```python
from build123d import *

# Parameters (mm, degrees)
SKETCH4_W           = 16.730770432
SKETCH4_H           = 61.894764582
SKETCH4_R           = 3.048230072
BOSS_EXTRUDE4_DEPTH = 10
BOSS_EXTRUDE5_DEPTH = 61.894764581
SKETCH6_R           = 3.22777379
CUT_EXTRUDE1_DEPTH  = 301.068940686
CUT_EXTRUDE2_START  = 17.78
SKETCH8_W           = 8.976833554
SKETCH8_H           = 8.976833554
CUT_EXTRUDE2_DEPTH  = 30.32
SKETCH9_R           = 3.75
CUT_EXTRUDE3_DEPTH  = 30.32
SKETCH10_R          = 8.1
CUT_EXTRUDE4_DEPTH  = 20


with BuildPart() as part:
    # Sketch4 → Boss-Extrude4 (new body)
    with BuildSketch(Plane.XY):
        with Locations((241.3, -38.1)):
            Rectangle(SKETCH4_W, SKETCH4_H)
        with Locations((241.3, -12.7)):
            Circle(SKETCH4_R, mode=Mode.SUBTRACT)
        with Locations((241.3, -38.1)):
            Circle(SKETCH4_R, mode=Mode.SUBTRACT)
        with Locations((241.3, -63.5)):
            Circle(SKETCH4_R, mode=Mode.SUBTRACT)
    extrude(amount=BOSS_EXTRUDE4_DEPTH)

    # Sketch5 → Boss-Extrude5 (add)
    with BuildSketch(Plane.XZ.offset(69.047382291)):
        Polygon((249.665385216, 10), (203.509422764, 131.615224448), (203.509422764, 151.462944604), (160.545206695, 151.462944604), (160.545206695, 127.74240556), (188.24848215, 127.74240556), (232.934614784, 10), align=None)
    extrude(amount=-BOSS_EXTRUDE5_DEPTH)

    # Sketch6 → Cut-Extrude1 (cut, through all)
    with BuildSketch(Plane(origin=(0, 0, 0), x_dir=(-1, 0, 0), z_dir=(0, 0, -1))):
        with Locations((-241.3, -63.5)):
            Circle(SKETCH6_R)
        with Locations((-241.3, -38.1)):
            Circle(SKETCH6_R)
        with Locations((-241.3, -12.7)):
            Circle(SKETCH6_R)
    extrude(amount=-CUT_EXTRUDE1_DEPTH, mode=Mode.SUBTRACT)

    # Sketch8 → Cut-Extrude2 (cut)
    with BuildSketch(Plane.XY.offset(CUT_EXTRUDE2_START)):
        with Locations((241.3, -63.5)):
            Rectangle(SKETCH8_W, SKETCH8_H)
        with Locations((241.3, -38.1)):
            Rectangle(SKETCH8_W, SKETCH8_H)
        with Locations((241.3, -12.7)):
            Rectangle(SKETCH8_W, SKETCH8_H)
    extrude(amount=CUT_EXTRUDE2_DEPTH, mode=Mode.SUBTRACT)

    # Sketch9 → Cut-Extrude3 (cut)
    with BuildSketch(Plane.XY.offset(151.462944604)):
        with Locations((182.02731473, -38.1)):
            Circle(SKETCH9_R)
    extrude(amount=-CUT_EXTRUDE3_DEPTH, mode=Mode.SUBTRACT)

    # Sketch10 → Cut-Extrude4 (cut)
    with BuildSketch(Plane.XY.offset(151.462944604)):
        with Locations((182.02731473, -38.1)):
            Circle(SKETCH10_R)
    extrude(amount=-CUT_EXTRUDE4_DEPTH, mode=Mode.SUBTRACT)


solid = part.part
```
Read the model definition and answer for the solid it produces. Units are mm, in the model's axes. A direction names the side the tool comes from. Round coordinates to 2 decimals unless told otherwise and drop trailing zeros. Write each loop counter-clockwise with the first axis right and the second up, starting at its lowest first coordinate (ties: lowest second). Pieces come first, ordered by that corner, then holes. Notation, with made-up numbers: (26.25, 38.25) - (77.25, 38.25) arc R22 ccw to (77.25, 74.25) - close; hole circle Ø3 at (-28.5, -34). An arc over 180 degrees is marked (long way). Use CSV: the item, a comma, the result in double quotes.
Q1. Find section D-D, the plane y = -63.5. Write down the section's boundary in (x, z).
Values:
outline,"(160.55, 127.74) - (188.25, 127.74) - (232.93, 10) - (232.93, 0) - (238.07, 0) - (238.07, 17.78) - (236.81, 17.78) - (236.81, 43.87) - (203.51, 131.62) - (203.51, 151.46) - (160.55, 151.46) - close; (244.53, 0) - (249.67, 0) - (249.67, 10) - (245.79, 20.22) - (245.79, 17.78) - (244.53, 17.78) - close"
Q2. Find section C-C, the plane z = 137.5. Write down the section's boundary in (x, y).
Values:
outline,"(160.55, -69.05) - (203.51, -69.05) - (203.51, -7.15) - (160.55, -7.15) - close; hole circle Ø16.2 at (182.03, -38.1)"
Q3. Each of these flat-tipped pins is pushed along its axis until it touches: pin 1 Ø3 at (y, z) = (-33, 126) entering from +X; pin 2 Ø12 at (x, y) = (182.03, -38.1) entering from -Z; pin 3 Ø3 at (y, z) = (-30.5, 93) entering from -X. Where does it stop, or does it pass through?
Values:
pin 1,"stops at x = 206.21"
pin 2,"stops at z = 127.74"
pin 3,"stops at x = 200.86"
Q4. Determine the mould class of faces 1 (the flat face through (210.279, -38.533, 69.695)), 2 (the flat face through (203.509, -39, 141)), 3 (the cylindrical face through (244.525, -12.558, 8.766)), 4 (the flat face through (208, -69.047, 87)) for opening direction X: +X half, -X half, draft (parallel to the pull), parting line (faces both ways), or undercut.
Values:
face 1,"-X half"
face 2,"+X half"
face 3,"undercut"
face 4,"draft"
Q5. Find section B-B, the plane x = 241.3. Write down the section's boundary in (y, z), then the cut area to 3 significant figures.
Values:
outline,"(-69.05, 0) - (-66.73, 0) - (-66.73, 17.78) - (-67.99, 17.78) - (-67.99, 32.04) - (-69.05, 32.04) - close; (-60.27, 0) - (-41.33, 0) - (-41.33, 17.78) - (-42.59, 17.78) - (-42.59, 32.04) - (-59.01, 32.04) - (-59.01, 17.78) - (-60.27, 17.78) - close; (-34.87, 0) - (-15.93, 0) - (-15.93, 17.78) - (-17.19, 17.78) - (-17.19, 32.04) - (-33.61, 32.04) - (-33.61, 17.78) - (-34.87, 17.78) - close; (-9.47, 0) - (-7.15, 0) - (-7.15, 32.04) - (-8.21, 32.04) - (-8.21, 17.78) - (-9.47, 17.78) - close"
area,"1,250 mm²"
Q6. A tool of negligible diameter and unlimited length cuts with its end or side. For faces 5 (the flat face through (174, -39, 127.742)), 6 (the flat face through (226.91, -38.53, 69.96)), 7 (the flat face through (238, -11, 17.78)), from which of +Z, -Z, +X, -X, +Y, -Y can it reach the whole face along a straight path? Write none if from no direction.
Values:
face 5,"-Z, -X, +Y, -Y"
face 6,"+Z, +X, +Y, -Y"
face 7,"+Z"
Q7. Find section A-A, the plane y = -38.1. Write down the section's boundary in (x, z), then the cut area to 3 significant figures.
Values:
outline,"(160.55, 127.74) - (178.28, 127.74) - (178.28, 131.46) - (173.93, 131.46) - (173.93, 151.46) - (160.55, 151.46) - close; (185.78, 127.74) - (188.25, 127.74) - (232.93, 10) - (232.93, 0) - (238.07, 0) - (238.07, 17.78) - (236.81, 17.78) - (236.81, 43.87) - (203.51, 131.62) - (203.51, 151.46) - (190.13, 151.46) - (190.13, 131.46) - (185.78, 131.46) - close; (244.53, 0) - (249.67, 0) - (249.67, 10) - (245.79, 20.22) - (245.79, 17.78) - (244.53, 17.78) - close"
area,"2,560 mm²"
Q8. Straight lines are drawn through the part: line 1 along Y through (x, z) = (241.3, 9); line 2 along Z through (x, y) = (176, -16); line 3 along X through (y, z) = (-65, 11). For each, find the intervals that lie inside material, in ascending order.
Values:
line 1,"y = -69.05 to -66.73, -60.27 to -41.33, -34.87 to -15.93, -9.47 to -7.15"
line 2,"z = 127.74 to 151.46"
line 3,"x = 232.56 to 238.44, 244.16 to 249.29"
